```python
from build123d import *

# Parameters (mm, degrees)
SKETCH1_W           = 185.42
SKETCH1_H           = 826.262
BOSS_EXTRUDE1_DEPTH = 2.54
CUT_EXTRUDE1_DEPTH  = 2.54
BOSS_EXTRUDE3_DEPTH = 2.54


with BuildPart() as part:
    # Sketch1 → Boss-Extrude1 (new body)
    with BuildSketch(Plane(origin=(0, 0, 0), x_dir=(1, 0, 0), z_dir=(0, 1, 0))):
        with Locations((2.261219512, -330.596487805)):
            Rectangle(SKETCH1_W, SKETCH1_H)
    extrude(amount=BOSS_EXTRUDE1_DEPTH)

    # Sketch2 → Cut-Extrude1 (cut)
    with BuildSketch(Plane(origin=(0, 2.54, 0), x_dir=(1, 0, 0), z_dir=(0, 1, 0))):
        Polygon((94.971219512, -743.727487805), (-90.448780488, -694.044348544), (-90.448780488, -743.727487805), align=None)
    extrude(amount=-CUT_EXTRUDE1_DEPTH, mode=Mode.SUBTRACT)

    # Sketch3 → Boss-Extrude3 (add)
    with BuildSketch(Plane.XZ):
        Polygon((-90.448780488, -82.534512195), (-90.448780488, -132.217651456), (94.971219512, -82.534512195), align=None)
    extrude(amount=-BOSS_EXTRUDE3_DEPTH)


solid = part.part
```
Verification items for the finished model (mm, model axes). Give positions to 0.01 mm unless a question says otherwise; leave off trailing zeros. Order: outer loops, then holes, each group sorted by start corner. A loop starts at its lowest first (then second) coordinate and runs counter-clockwise, first axis right, second up. Notation, with made-up numbers: (-31.75, 89.25) -> (10.25, 89.25) arc R10 ccw to (10.25, 102.25) -> close; hole circle Ø1 at (-16.5, -16.5). An arc over 180 degrees is marked (long way). Use a Markdown table: item, result.
1) Material ranges on probe 1 along Z at (x, y) = (18, 0.2); probe 2 along Z at (x, y) = (-72.5, 2.1), recorded low to high.
Results:
| item | result |
|---|---|
| probe 1 | -103.16 to 723.1 |
| probe 2 | -127.41 to 698.85 |
2) Section check B-B, the plane x = 33. Record the boundary of the cut face in (y, z).
Results:
| item | result |
|---|---|
| outline | (0, -99.14) -> (2.54, -99.14) -> (2.54, 727.12) -> (0, 727.12) -> close |
3) Section check A-A, the plane y = 1.55. Record the boundary of the cut face in (x, z).
Results:
| item | result |
|---|---|
| outline | (-90.45, -132.22) -> (94.97, -82.53) -> (94.97, 743.73) -> (-90.45, 694.04) -> close |
4) Depth check by flat-ended pin: pin 1 Ø1 at (x, y) = (-30.5, 0.5) entering from -Z. Enter the tip coordinate at first touch or a pass-through.
Results:
| item | result |
|---|---|
| pin 1 | z = -116.29 |
